from build123d import *

# Parameters (mm, degrees)
CROQUIS1_W              = 27
CROQUIS1_H              = 43
SALIENTE_EXTRUIR1_DEPTH = 4.5
CROQUIS2_R              = 3.5
SALIENTE_EXTRUIR2_DEPTH = 3
CROQUIS3_R              = 1.5
CORTAR_EXTRUIR1_DEPTH   = 5


with BuildPart() as part:
    # Croquis1 → Saliente-Extruir1 (new, symmetric)
    with BuildSketch(Plane.XY):
        Rectangle(CROQUIS1_W, CROQUIS1_H)
    extrude(amount=SALIENTE_EXTRUIR1_DEPTH, both=True)

    # Croquis2 → Saliente-Extruir2 (add)
    with BuildSketch(Plane(origin=(13.5, 0, 0), x_dir=(0, 0, -1), z_dir=(1, 0, 0))):
        with Locations(Location((0, -14.5, 0), (0, 0, 180))):
            Circle(CROQUIS2_R)
    saliente_extruir2 = extrude(amount=SALIENTE_EXTRUIR2_DEPTH)

    # Croquis3 → Cortar-Extruir1 (cut)
    with BuildSketch(Plane(origin=(16.5, 0, 0), x_dir=(0, 0, -1), z_dir=(1, 0, 0))):
        with Locations((0, -14.5)):
            Circle(CROQUIS3_R)
    cortar_extruir1 = extrude(amount=-CORTAR_EXTRUIR1_DEPTH, mode=Mode.SUBTRACT)

    # Simetría2: Saliente-Extruir2, Cortar-Extruir1 across plane
    add(saliente_extruir2.mirror(Plane(origin=(0, 0, 0), x_dir=(0, 0, 1), z_dir=(1, 0, 0))))
    add(cortar_extruir1.mirror(Plane(origin=(0, 0, 0), x_dir=(0, 0, 1), z_dir=(1, 0, 0))), mode=Mode.SUBTRACT)


solid = part.part
Check sheet for the modelled part. Datum: model origin and axes. Units: mm. A direction names the side the tool comes from. Give positions to 0.01 mm unless a question says otherwise; leave off trailing zeros. Write each loop counter-clockwise with the first axis right and the second up, starting at its lowest first coordinate (ties: lowest second). Pieces come first, ordered by that corner, then holes. Notation, with made-up numbers: (12.5, -11.5) -> (56.5, -11.5) arc R14 cw to (56.5, -0.5) -> close; hole circle Ø8 at (32.25, -35.5). An arc over 180 degrees is marked (long way). Write item = value, one per line.
Item 1: Sectioned sample at D-D on z = -2.75. Record the boundary of the cut face in (x, y), and give its area (3 significant figures).
Output:
outline = (-16.5, -16.67) -> (-13.5, -16.67) -> (-13.5, -21.5) -> (13.5, -21.5) -> (13.5, -16.67) -> (16.5, -16.67) -> (16.5, -12.33) -> (13.5, -12.33) -> (13.5, 21.5) -> (-13.5, 21.5) -> (-13.5, -12.33) -> (-16.5, -12.33) -> close
area = 1,190 mm^2
Item 2: Gauge pin test, flat ends, axial feed: pin 1 (3 mm diameter, centred on y = -6, z = 0, fed in from -X); pin 2 (1.8 mm diameter, centred on y = -14.5, z = 0, fed in from -X). Record the tip position at first contact, or that the pin passes through.
Output:
pin_1 = -13.5
pin_2 = -11.5
Item 3: Sectioned sample at B-B on y = -9.5. Record the boundary of the cut face in (x, z), and give its area (3 significant figures).
Output:
outline = (-13.5, -4.5) -> (13.5, -4.5) -> (13.5, 4.5) -> (-13.5, 4.5) -> close
area = 243 mm^2
Item 4: Tool access check on faces 5 (the cylindrical face through (14.979, -11.083, -0.759)), 6 (the cylindrical face through (-14, -16, 0)), 7 (the flat face through (0, -21.5, 0)). Record the directions out of +Z, -Z, +X, -X, +Y, -Y that give a thin tool (end or side, any length) a straight path to the whole face; none if there is none.
Output:
face_5 = +X
face_6 = -X
face_7 = +Z, -Z, +X, -X, -Y
Item 5: Sectioned sample at C-C on z = 2. Record the boundary of the cut face in (x, y).
Output:
outline = (-16.5, -17.37) -> (-13.5, -17.37) -> (-13.5, -21.5) -> (13.5, -21.5) -> (13.5, -17.37) -> (16.5, -17.37) -> (16.5, -11.63) -> (13.5, -11.63) -> (13.5, 21.5) -> (-13.5, 21.5) -> (-13.5, -11.63) -> (-16.5, -11.63) -> close
Item 6: Scan lines: probe 1 along Y at (x, z) = (13, 0); probe 2 along Y at (x, z) = (-14.1, 0); probe 3 along X at (y, z) = (13.5, -4). Record each from-to range of solid material in increasing order. Write a range as from..to.
Output:
probe_1 = -21.5..-16, -13..21.5
probe_2 = -18..-16, -13..-11
probe_3 = -13.5..13.5
Item 7: Sectioned sample at A-A on z = 0. Record the boundary of the cut face in (x, y).
Output:
outline = (-16.5, -18) -> (-13.5, -18) -> (-13.5, -21.5) -> (13.5, -21.5) -> (13.5, -18) -> (16.5, -18) -> (16.5, -16) -> (11.5, -16) -> (11.5, -13) -> (16.5, -13) -> (16.5, -11) -> (13.5, -11) -> (13.5, 21.5) -> (-13.5, 21.5) -> (-13.5, -11) -> (-16.5, -11) -> (-16.5, -13) -> (-11.5, -13) -> (-11.5, -16) -> (-16.5, -16) -> close
Item 8: Release check for a two-part mould opening along Y. For faces 1 (the flat face through (-13.5, 0, 0)), 2 (the cylindrical face through (14, -16, 0)), 3 (the cylindrical face through (-14.979, -11.083, -0.759)), 4 (the flat face through (0, 21.5, 0)) record: +Y half, -Y half, draft (parallel to the pull), parting line (faces both ways), or undercut.
Output:
face_1 = draft
face_2 = undercut
face_3 = parting line
face_4 = +Y half
